```python
from build123d import *

# Parameters (mm, degrees)
SKETCH1_R               = 10
BOSS_EXTRUDE1_DEPTH     = 40
SKETCH2_R               = 20
BOSS_EXTRUDE2_DEPTH     = 3
CIRPATTERN1_COUNT       = 4
CUT_EXTRUDE1_DEPTH      = 49.989794856
CUT_EXTRUDE1_DEPTH_BACK = 49.989794856
M6_TAPPED_HOLE1_D       = 5
M6_TAPPED_HOLE1_DEPTH   = 10
M6_TAPPED_HOLE1_TIP     = 1.502151548


with BuildPart() as part:
    # Sketch1 → Boss-Extrude1 (new body)
    with BuildSketch(Plane(origin=(0, 0, 0), x_dir=(1, 0, 0), z_dir=(0, 1, 0))):
        with Locations(Location((0, 0, 0), (0, 0, 270))):
            Circle(SKETCH1_R)
    extrude(amount=BOSS_EXTRUDE1_DEPTH)

    # Sketch2 → Boss-Extrude2 (add)
    with BuildSketch(Plane.XZ):
        with Locations(Location((0, 0, 0), (0, 0, 270))):
            Circle(SKETCH2_R)
    extrude(amount=-BOSS_EXTRUDE2_DEPTH)

    # Sketch3 → CSK for M3 Countersunk Flat Head Screw1 (revolve, cut)
    with BuildSketch(Plane(origin=(0, 3, -15), x_dir=(0, 0, 1), z_dir=(1, 0, 0))):
        Polygon((0, 0), (0, 3), (1.7, 3), (1.7, 1.45), (3.15, 0), align=None)
    csk_for_m3_countersunk_flat_head_screw1 = revolve(axis=Axis((0, 9.35, -15), (0, -1, 0)), mode=Mode.SUBTRACT)

    # CirPattern1: CSK for M3 Countersunk Flat Head Screw1 ×4 about axis
    cirpattern1_axis = Axis((0, 0, 0), (0, 1, 0))
    for i in range(1, CIRPATTERN1_COUNT):
        add(csk_for_m3_countersunk_flat_head_screw1.rotate(cirpattern1_axis, i * 360 / CIRPATTERN1_COUNT), mode=Mode.SUBTRACT)

    # Sketch5 → Cut-Extrude1 (cut, two sides: drawn at the far end of the back side and taken through both)
    with BuildSketch(Plane.XY.offset(-CUT_EXTRUDE1_DEPTH_BACK)):
        Polygon((-10, 40), (10, 40), (-10, 20), align=None)
    extrude(amount=CUT_EXTRUDE1_DEPTH + CUT_EXTRUDE1_DEPTH_BACK, mode=Mode.SUBTRACT)

    # M6 Tapped Hole1
    with Locations(Plane(origin=(-15, 15, 0), x_dir=(0.7071067811865475, 0.7071067811865477, 0), z_dir=(-0.7071067811865477, 0.7071067811865475, 0))):
        with Locations((21.213203436, 0)):
            Hole(M6_TAPPED_HOLE1_D / 2, depth=M6_TAPPED_HOLE1_DEPTH)
            with Locations((0, 0, -(M6_TAPPED_HOLE1_DEPTH + M6_TAPPED_HOLE1_TIP / 2))):  # 118° drill point
                Cone(0, M6_TAPPED_HOLE1_D / 2, M6_TAPPED_HOLE1_TIP, mode=Mode.SUBTRACT)


solid = part.part
```
Model file for the job. Use its own axes, mm. A direction names the side the tool comes from. Round coordinates to 2 decimals unless told otherwise and drop trailing zeros. Write each loop counter-clockwise with the first axis right and the second up, starting at its lowest first coordinate (ties: lowest second). Pieces come first, ordered by that corner, then holes. Notation, with made-up numbers: M 43.5,57.5 L 99.5,57.5 A29 ccw 99.5,81.5 Z; hole C -10,53.25 d9. An arc over 180 degrees is marked long. Put each result on its own line as item: value.
Item 1: Flat gauge pins, fed straight in: P1, Ø10, axis at y = 13.5, z = -5, coming from the -X side; P2, Ø8, axis at x = -4, y = 25.5, coming from the +Z side; P3, Ø3, axis at x = 4.5, y = 31, coming from the -Z side; P4, Ø2, axis at x = 0, z = -15, coming from the +Y side. Where does each tip first touch, or does it go through?
Responses:
P1: x = -10
P2: z = 10
P3: z = -9.54
P4: through
Item 2: Cut at D-D (z = -4). List the corners of the cut face in (x, y), and give its area (3 significant figures).
Responses:
outline: M -19.6,0 L 19.6,0 L 19.6,3 L 9.17,3 L 9.17,39.17 L -9.17,20.83 L -9.17,3 L -19.6,3 Z
area: 612 mm²
Item 3: Mould opens along Z. For faces 4 (the cylindrical face through (13.38, 0.79, -0.51)), 5 (the flat face through (9, 3, 5)), 6 (the cylindrical face through (-19.524, 1.479, 4.336)) say: +Z half, -Z half, draft (parallel to the pull), parting line (faces both ways), or undercut.
Responses:
face 4: undercut
face 5: draft
face 6: parting line
Item 4: Tool access for faces 1 (the conical face through (7.642, 21.745, -0.019)), 2 (the flat face through (-2, 28, 0)), 3 (the cylindrical face through (9.915, 17.13, -1.302)): list every direction of +Z, -Z, +X, -X, +Y, -Y with a clear straight run to the whole face (end or side of a thin tool).
Responses:
face 1: none
face 2: +Z, -Z, -X, +Y
face 3: +Y
Item 5: Cut at A-A (x = -15). List the corners of the cut face in (y, z).
Responses:
outline: M 0,-13.23 L 3,-13.23 L 3,-3.15 L 1.55,-1.7 L 0,-1.7 Z; M 0,1.7 L 1.55,1.7 L 3,3.15 L 3,13.23 L 0,13.23 Z
Item 6: Probe L1, parallel to Y at x = -12, z = 15; L2, parallel to X at y = 27, z = -5.5; L3, parallel to Y at x = -7, z = 6. List the from-to ranges inside material, lowest first. Write a range as from..to.
Responses:
L1: 0..3
L2: -3..8.35
L3: 0..23
Item 7: Cut at B-B (z = 15). List the corners of the cut face in (x, y), and give its area (3 significant figures).
Responses:
outline: M -13.23,0 L -1.7,0 L -1.7,1.55 L -3.15,3 L -13.23,3 Z; M 1.7,0 L 13.23,0 L 13.23,3 L 3.15,3 L 1.7,1.55 Z
area: 67.1 mm²
Item 8: Cut at C-C (x = -8). List the corners of the cut face in (y, z).
Responses:
outline: M 0,-18.33 L 3,-18.33 L 3,-6 L 22,-6 L 22,6 L 3,6 L 3,18.33 L 0,18.33 Z
